from build123d import *

# Parameters (mm, degrees)
F0_W                 = 130
F0_H                 = 45
F1_DEPTH             = 12
F2_R                 = 5
F5_D                 = 5.5
F5_CBORE_D           = 9.75
F5_CBORE_DEPTH       = 6
F5_ON_F4_D           = 5.5
F5_ON_F4_CBORE_D     = 9.75
F5_ON_F4_CBORE_DEPTH = 6
F6_T1_DEPTH          = 65.7168298797
F7_R                 = 2.75
F8_DEPTH             = 2


# Not quite as in the source:
# - a fillet or chamfer that OpenCascade refuses, or shapes differently, is made with other operations: its cross-section is extruded or revolved along the edge and cut away or added


with BuildPart() as f1:
    # F0 (on Top) → F1 (new body)
    with BuildSketch(Plane.XY):
        Rectangle(F0_W, F0_H)
    extrude(amount=F1_DEPTH)

    # F2
    f2_edges = [f1.edges().sort_by_distance(p)[0] for p in [
        (65, -22.5, 6),
        (-65, -22.5, 6),
    ]]
    fillet(f2_edges, radius=F2_R)

    # F5 (through all)
    with Locations(Plane.XY.offset(12)):
        with Locations((-57.5, -5), (-57.5, 15), (57.5, -5), (57.5, 15), (-42.5, -17.5), (42.5, -17.5)):
            CounterBoreHole(F5_D / 2, F5_CBORE_D / 2, F5_CBORE_DEPTH)

    # F5 on F4 (through all)
    with Locations(Plane.XY.offset(12)):
        with Locations((-20, 5.5), (20, 5.5)):
            CounterBoreHole(F5_ON_F4_D / 2, F5_ON_F4_CBORE_D / 2, F5_ON_F4_CBORE_DEPTH)

    # F6: chamfer of 5 on 2 edges, made by hand

    # F6_s2 → F6_t1 (cut)
    with BuildSketch(Plane.XZ.offset(-35.3584149398)):
        Polygon((-60, 12), (-65, 7), (-65, 12), align=None)
        Polygon((60, 12), (65, 7), (65, 12), align=None)
    extrude(amount=F6_T1_DEPTH, mode=Mode.SUBTRACT)

    # F7 (on face) → F8 (cut)
    with BuildSketch(Plane(origin=(0, 0, 0), x_dir=(1, 0, 0), z_dir=(0, 0, -1))):
        with BuildLine():
            Line((-18.3303027798, -22.5), (18.3303027798, -22.5))
            ThreePointArc((18.3303027798, -22.5), (25, -5.5), (18.3303027798, 11.5))
            Line((18.3303027798, 11.5), (-18.3303027798, 11.5))
            ThreePointArc((-18.3303027798, 11.5), (-25, -5.5), (-18.3303027798, -22.5))
        make_face()
        with Locations((-20, -5.5)):
            Circle(F7_R, mode=Mode.SUBTRACT)
        with Locations((20, -5.5)):
            Circle(F7_R, mode=Mode.SUBTRACT)
    extrude(amount=-F8_DEPTH, mode=Mode.SUBTRACT)


solid = f1.part
The model under review builds one solid part; all positions refer to its coordinate system, in mm. A direction names the side the tool comes from. Give positions to 0.01 mm unless a question says otherwise; leave off trailing zeros. Order: outer loops, then holes, each group sorted by start corner. A loop starts at its lowest first (then second) coordinate and runs counter-clockwise, first axis right, second up. Notation, with made-up numbers: M -8.5,49.25 L 5.5,49.25 A30 ccw 5.5,74.25 Z; hole C -17.75,87 d1. An arc over 180 degrees is marked long. Use one line per item in the form item = value. Start each with the question number.
Item 1: We need section C-C on y = 15. Give the boundary of the cut face in (x, z) (3 decimals), plus the area to 3 significant figures.
Item 2: Insertion check: pin 1 Ø3 at (y, z) = (4.5, 7.5) entering from +X; pin 2 Ø8 at (x, y) = (-43, -17) entering from +Z; pin 3 Ø1 at (x, y) = (-11.5, -4) entering from -Z. Each pin has a flat end and moves straight along its axis. Give the tip position at first contact, or say it passes through.
Item 3: To check wall thickness, follow line 1 along Y through (x, z) = (-57.5, 4.85); line 2 along X through (y, z) = (15, 7.4) (3 decimals); line 3 along X through (y, z) = (19, 8.5). State the ranges of each line that lie inside material, in increasing order. Write a range as from..to.
Item 4: We need section A-A on x = -42.5. Give the boundary of the cut face in (y, z) (3 decimals).
Item 5: The part is to be moulded in two halves that separate along X. For faces 3 (the flat face through (-40, -20, 6)), 4 (the flat face through (-65, 2, 3)), 5 (the flat face through (-1, 0, 12)), say which applies: pulls with the +X half, pulls with the -X half, needs draft (parallel to the pull), parting line crosses it, or undercut.
Item 6: For faces 1 (the cylindrical face through (52.63, 15.21, 9.04)), 2 (the cylindrical face through (-54.753, 15.121, 2.958)), list the 3-axis set-ups (+Z, -Z, +X, -X, +Y, -Y) from which the entire face can be reached by the end or side of a thin tool; tool diameter is ignored.
Item 7: We need section B-B on x = -57.5. Give the boundary of the cut face in (y, z) (3 decimals).
Item 8: We need section D-D on x = -20. Give the boundary of the cut face in (y, z) (3 decimals).
Completed:
q1.outline = M -65,0 L -60.25,0 L -60.25,6 L -62.375,6 L -62.375,9.625 L -65,7 Z; M -54.75,0 L -23.125,0 L -23.125,2 L 23.125,2 L 23.125,0 L 54.75,0 L 54.75,6 L 52.625,6 L 52.625,12 L -52.625,12 L -52.625,6 L -54.75,6 Z; M 60.25,0 L 65,0 L 65,7 L 62.375,9.625 L 62.375,6 L 60.25,6 Z
q1.area = 1,270 mm²
q2.pin_1 = 65
q2.pin_2 = 6
q2.pin_3 = 2
q3.line_1 = -22.5..-7.75, -2.25..12.25, 17.75..22.5
q3.line_2 = -64.6..-62.375, -52.625..52.625, 62.375..64.6
q3.line_3 = -63.5..-60.29, -54.71..54.71, 60.29..63.5
q4.outline = M -22.5,0 L -20.25,0 L -20.25,6 L -22.375,6 L -22.375,12 L -22.5,12 Z; M -14.75,0 L 22.5,0 L 22.5,12 L -12.625,12 L -12.625,6 L -14.75,6 Z
q5.face_3 = undercut
q5.face_4 = pulls with the -X half
q5.face_5 = needs draft
q6.face_1 = +Z
q6.face_2 = +Z, -Z
q7.outline = M -22.5,0 L -7.75,0 L -7.75,6 L -9.875,6 L -9.875,12 L -22.5,12 Z; M -2.25,0 L 12.25,0 L 12.25,6 L 10.125,6 L 10.125,12 L -0.125,12 L -0.125,6 L -2.25,6 Z; M 17.75,0 L 22.5,0 L 22.5,12 L 19.875,12 L 19.875,6 L 17.75,6 Z
q8.outline = M -22.5,0 L -9.5,0 L -9.5,2 L 2.75,2 L 2.75,6 L 0.625,6 L 0.625,12 L -22.5,12 Z; M 8.25,2 L 20.5,2 L 20.5,0 L 22.5,0 L 22.5,12 L 10.375,12 L 10.375,6 L 8.25,6 Z
